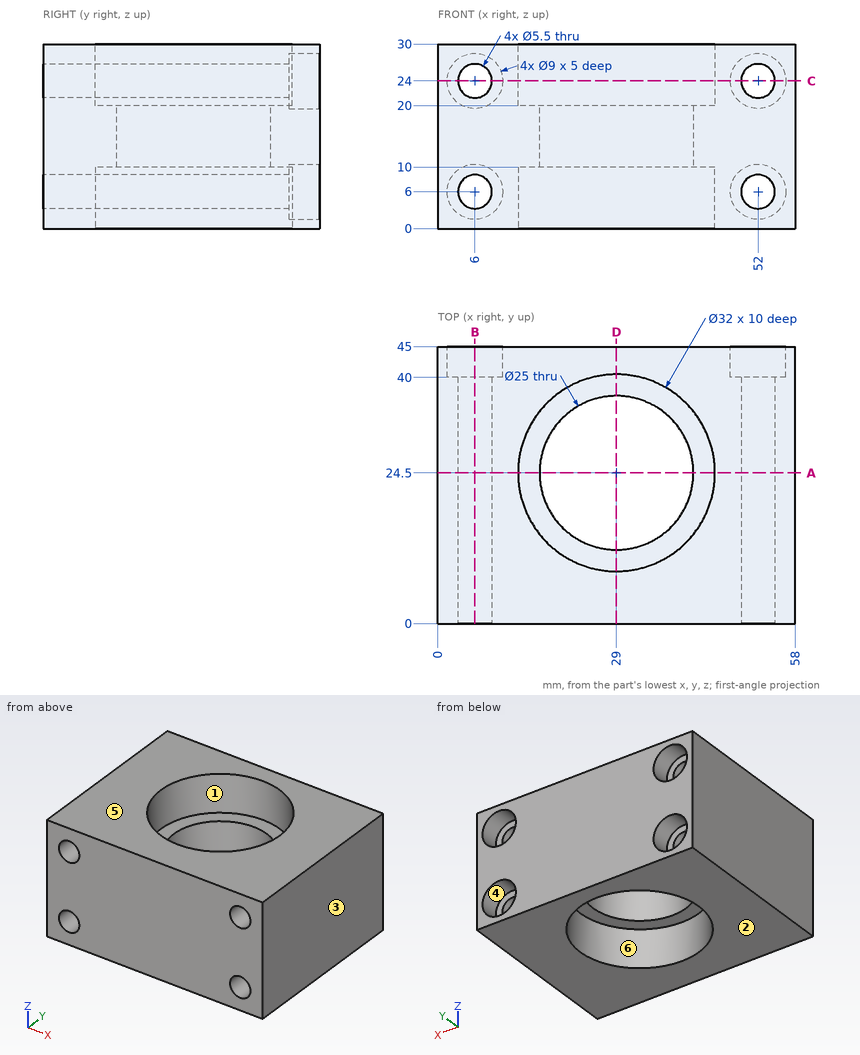
Answer from the drawing. Dimensions are ordinates in mm from the lowest x, y and z of the part. A direction names the side the tool comes from. Round coordinates to 2 decimals unless told otherwise and drop trailing zeros. Write each loop counter-clockwise with the first axis right and the second up, starting at its lowest first coordinate (ties: lowest second). Pieces come first, ordered by that corner, then holes.
1. The part is cut by section A-A, the plane y = 24.5. Determine the outline of the cut face in (x, z).
2. Determine the mould class of the marked faces 1, 2 and 3 for opening direction X: pulls with the +X half, pulls with the -X half, needs draft (parallel to the pull), parting line crosses it, or undercut.
3. The part is cut by section C-C, the plane z = 24. Determine the outline of the cut face in (x, y).
4. Given pin 1 Ø7 at (x, z) = (52, 24) entering from +Y; pin 2 Ø3 at (x, y) = (16.5, 30.5) entering from +Z; pin 3 Ø9.5 at (x, y) = (35, 22) entering from -Z, each flat-ended and moving along its own axis, determine where each tip first touches the part or whether it passes through.
5. The part is cut by section B-B, the plane x = 6. Determine the outline of the cut face in (y, z).
6. Which of the six approach directions +Z, -Z, +X, -X, +Y, -Y give full straight-line access (tool end or side, diameter ignored) to the marked faces 4, 5 and 6?
7. The part is cut by section D-D, the plane x = 29. Determine the outline of the cut face in (y, z).
8. Straight lines are drawn through the part: L1, parallel to Z at x = 52, y = 43; L2, parallel to X at y = 13, z = 24; L3, parallel to X at y = 17, z = 6. For each, find the intervals that lie inside material, in ascending order.
Values:
1. outline: (0, 0) - (13, 0) - (13, 10) - (16.5, 10) - (16.5, 20) - (13, 20) - (13, 30) - (0, 30) - close; (41.5, 10) - (45, 10) - (45, 0) - (58, 0) - (58, 30) - (45, 30) - (45, 20) - (41.5, 20) - close; hole circle Ø5.5 at (6, 6); hole circle Ø5.5 at (6, 24); hole circle Ø5.5 at (52, 6); hole circle Ø5.5 at (52, 24)
2. face 1: undercut
2. face 2: needs draft
2. face 3: pulls with the +X half
3. outline: (0, 0) - (3.25, 0) - (3.25, 40) - (1.5, 40) - (1.5, 45) - (0, 45) - close; (8.75, 0) - (49.25, 0) - (49.25, 40) - (47.5, 40) - (47.5, 45) - (10.5, 45) - (10.5, 40) - (8.75, 40) - close; (54.75, 0) - (58, 0) - (58, 45) - (56.5, 45) - (56.5, 40) - (54.75, 40) - close; hole circle Ø32 at (29, 24.5)
4. pin 1: stops at y = 40
4. pin 2: stops at z = 20
4. pin 3: passes through
5. outline: (0, 0) - (45, 0) - (45, 1.5) - (40, 1.5) - (40, 3.25) - (0, 3.25) - close; (0, 8.75) - (40, 8.75) - (40, 10.5) - (45, 10.5) - (45, 19.5) - (40, 19.5) - (40, 21.25) - (0, 21.25) - close; (0, 26.75) - (40, 26.75) - (40, 28.5) - (45, 28.5) - (45, 30) - (0, 30) - close
6. face 4: +Y
6. face 5: +Z, +X, -X, +Y, -Y
6. face 6: -Z
7. outline: (0, 0) - (8.5, 0) - (8.5, 10) - (12, 10) - (12, 20) - (8.5, 20) - (8.5, 30) - (0, 30) - close; (37, 10) - (40.5, 10) - (40.5, 0) - (45, 0) - (45, 30) - (40.5, 30) - (40.5, 20) - (37, 20) - close
8. L1: z = 0 to 1.5, 10.5 to 19.5, 28.5 to 30
8. L2: x = 0 to 3.25, 8.75 to 17.88, 40.12 to 49.25, 54.75 to 58
8. L3: x = 0 to 3.25, 8.75 to 14.87, 43.13 to 49.25, 54.75 to 58
